```python
from build123d import *

# Parameters (mm, degrees)
BOSS_EXTRUDE1_DEPTH = 9.5
SKETCH4_R           = 0.785
SKETCH4_R_2         = 0.51
BOSS_EXTRUDE2_DEPTH = 12


with BuildPart() as part:
    # Sketch1 → Boss-Extrude1 (new body)
    with BuildSketch(Plane(origin=(0, 0, 0), x_dir=(1, 0, 0), z_dir=(0, 1, 0))):
        Polygon((-31.1, 23.1), (-33.1, 21.1), (-33.1, 0), (0, 0), (0, 23.1), align=None)
    extrude(amount=BOSS_EXTRUDE1_DEPTH)

    # Sketch4 → Boss-Extrude2 (add)
    with BuildSketch(Plane(origin=(0, 9.5, 0), x_dir=(1, 0, 0), z_dir=(0, 1, 0))):
        with Locations(Location((-2.7, 19.14, 0), (0, 0, 270))):
            Circle(SKETCH4_R)
        with Locations((-2.7, 19.14)):
            Circle(SKETCH4_R_2, mode=Mode.SUBTRACT)
        with Locations((-2.7, 19.14)):
            Circle(SKETCH4_R_2)
        with Locations(Location((-2.7, 15.33, 0), (0, 0, 270))):
            Circle(SKETCH4_R_2)
        with Locations(Location((-2.7, 3.9, 0), (0, 0, 270))):
            Circle(SKETCH4_R)
        with Locations((-2.7, 3.9)):
            Circle(SKETCH4_R_2, mode=Mode.SUBTRACT)
        with Locations((-2.7, 3.9)):
            Circle(SKETCH4_R_2)
        with Locations(Location((-2.7, 7.71, 0), (0, 0, 270))):
            Circle(SKETCH4_R_2)
        with Locations(Location((-2.7, 11.52, 0), (0, 0, 270))):
            Circle(SKETCH4_R_2)
        with Locations(Location((-30.64, 3.9, 0), (0, 0, 270))):
            Circle(SKETCH4_R_2)
        with Locations(Location((-30.64, 19.14, 0), (0, 0, 270))):
            Circle(SKETCH4_R_2)
        with Locations(Location((-30.64, 11.52, 0), (0, 0, 270))):
            Circle(SKETCH4_R_2)
    extrude(amount=-BOSS_EXTRUDE2_DEPTH)


solid = part.part
```
Source: CAD feature listing. Evaluate the final solid. Frame: model axes, mm. A direction names the side the tool comes from. Give positions to 0.01 mm unless a question says otherwise; leave off trailing zeros. Write each loop counter-clockwise with the first axis right and the second up, starting at its lowest first coordinate (ties: lowest second). Pieces come first, ordered by that corner, then holes. Notation, with made-up numbers: (45.5, 40.5) - (80.5, 40.5) arc R20 cw to (80.5, 52.5) - close; hole circle Ø10 at (-24.75, -23). An arc over 180 degrees is marked (long way). One line per item, written item: value. Start each with the question number.
Q1. Section query D-D, the plane z = -3.9. Return the cut outline in (x, y) (3 decimals), then the cut area to 3 significant figures.
Q2. Section query B-B, the plane z = -15.33. Return the cut outline in (x, y).
Q3. Section query A-A, the plane y = -1.5. Return the cut outline in (x, z) (3 decimals).
Q4. Section query C-C, the plane x = -2.7. Return the cut outline in (y, z) (3 decimals).
Q5. Draft query along X for faces 1 (the face through (-3, -2.5, -4)), 2 (the face through (-30.134, -1.232, -11.586)), 3 (the face through (-32.1, 4.7, -22.1)). Return one class per face: +X half, -X half, draft (parallel to the pull), parting line (faces both ways), or undercut.
Q6. Material intervals for probe 1 along Z at (x, y) = (-2.5, -2); probe 2 along Y at (x, z) = (-23, -16.5); probe 3 along X at (y, z) = (2, -22), sorted ascending. Write a range as from..to.
Q7. Set-up query: faces 4 (the face through (-2.665, -1.232, -4.684)), 5 (the face through (-3, -2.5, -19)). Return all of +Z, -Z, +X, -X, +Y, -Y with unobstructed straight access to the full face (end or side cutting, diameter ignored); none if empty.
Q8. First-contact query: pin 1 Ø3 at (x, z) = (-18, -19) entering from -Y. Flat tip, straight axial feed; report the tip coordinate or a pass-through.
Answer:
1. outline: (-33.1, 0) - (-31.15, 0) - (-31.15, -2.5) - (-30.13, -2.5) - (-30.13, 0) - (-3.485, 0) - (-3.485, -2.5) - (-1.915, -2.5) - (-1.915, 0) - (0, 0) - (0, 9.5) - (-33.1, 9.5) - close
1. area: 321 mm2
2. outline: (-33.1, 0) - (-3.21, 0) - (-3.21, -2.5) - (-2.19, -2.5) - (-2.19, 0) - (0, 0) - (0, 9.5) - (-33.1, 9.5) - close
3. outline: circle Ø1.02 at (-30.64, -19.14); circle Ø1.02 at (-30.64, -11.52); circle Ø1.02 at (-30.64, -3.9); circle Ø1.57 at (-2.7, -19.14); circle Ø1.57 at (-2.7, -3.9); circle Ø1.02 at (-2.7, -15.33); circle Ø1.02 at (-2.7, -11.52); circle Ø1.02 at (-2.7, -7.71)
4. outline: (-2.5, -19.925) - (0, -19.925) - (0, -23.1) - (9.5, -23.1) - (9.5, 0) - (0, 0) - (0, -3.115) - (-2.5, -3.115) - (-2.5, -4.685) - (0, -4.685) - (0, -7.2) - (-2.5, -7.2) - (-2.5, -8.22) - (0, -8.22) - (0, -11.01) - (-2.5, -11.01) - (-2.5, -12.03) - (0, -12.03) - (0, -14.82) - (-2.5, -14.82) - (-2.5, -15.84) - (0, -15.84) - (0, -18.355) - (-2.5, -18.355) - close
5. face 1: draft
5. face 2: undercut
5. face 3: -X half
6. probe 1: z = -19.9..-18.38, -15.8..-14.86, -11.99..-11.05, -8.18..-7.24, -4.66..-3.14
6. probe 2: y = 0..9.5
6. probe 3: x = -32.2..0
7. face 4: -Y
7. face 5: +Z, -Z, +X, -X, -Y
8. pin 1: stops at y = 0
